Read the model definition and answer for the solid it produces. Units are mm, in the model's axes. Face numbers are marked on the shaded views. A direction names the side the tool comes from. Round coordinates to 2 decimals unless told otherwise and drop trailing zeros. Order: outer loops, then holes, each group sorted by start corner. A loop starts at its lowest first (then second) coordinate and runs counter-clockwise, first axis right, second up. Notation, with made-up numbers: (-24, 36.25) -> (12, 36.25) arc R17 ccw to (12, 67.25) -> close; hole circle Ø4 at (80.25, 17.25). An arc over 180 degrees is marked (long way). One line per item, written item: value. Start each with the question number.
1. Section C-C (z = 11.5) is taken. Give the vertices of the cut face in (x, y).
2. Flat-ended cylindrical pins translate along their axes: pin 1 Ø4.5 at (x, y) = (0, 10.5) entering from -Z; pin 2 Ø4.5 at (x, z) = (-3, 17.5) entering from -Y; pin 3 Ø4.5 at (x, z) = (-1.5, 7.5) entering from +Y. Find the tip coordinate at first contact, or state that the pin passes through.
3. Consider line 1 (X direction, y = 10.5, z = 35.05) (3 decimals); line 2 (Z direction, x = -7, y = -11.5); line 3 (Y direction, x = -0.25, z = 19). Determine where each line is inside the solid, lowest interval first.
4. Section B-B (x = 0) is taken. Give the vertices of the cut face in (y, z) (3 decimals).
5. Section A-A (y = 10.5) is taken. Give the vertices of the cut face in (x, z) (3 decimals), then the cut area to 3 significant figures.
6. For the marked faces 1, 2, 3 and 4, determine the directions among +Z, -Z, +X, -X, +Y, -Y from which every point of the face is accessible in a straight line to the end or side of a thin tool.
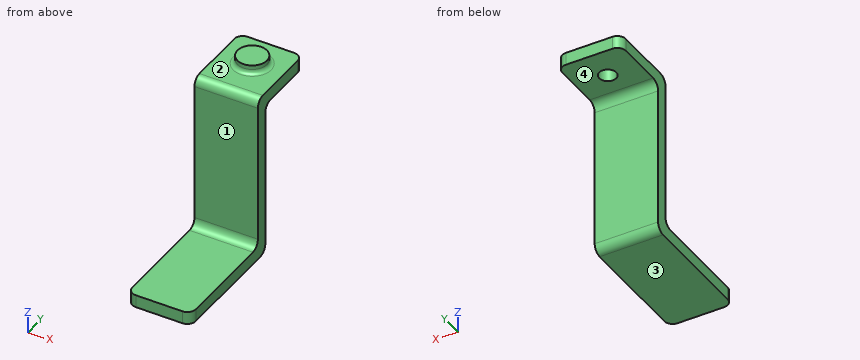
from build123d import *

# Parameters (mm, degrees)
EXTRUDE_1_DEPTH      = 7.5
EXTRUDE_1_DEPTH_BACK = 7.5
FILLET_1_R           = 2
SKETCH_2_R           = 3.5
EXTRUDE_3_DEPTH      = 2
SKETCH_4_R           = 2.025
CUT_EXTRUDE_1_DEPTH  = 4
FILLET_2_R           = 1


with BuildPart() as part:
    # Sketch 1 → Extrude 1 (new, two sides: drawn at the far end of the back side and taken through both)
    with BuildSketch(Plane(origin=(0, 0, 0), x_dir=(0, 0, -1), z_dir=(1, 0, 0)).offset(-EXTRUDE_1_DEPTH_BACK)):
        Polygon((-34, 18), (-34, 3), (3, 3), (3, -27), (0, -27), (0, 0), (-37, 0), (-37, 18), align=None)
    extrude(amount=EXTRUDE_1_DEPTH + EXTRUDE_1_DEPTH_BACK)

    # Fillet 1
    fillet_1_edges = [part.edges().sort_by_distance(p)[0] for p in [
        (0, 3, 34),
        (0, 3, -3),
        (0, 0, 0),
        (0, 0, 37),
        (-7.5, -27, -1.5),
        (7.5, 18, 35.5),
        (7.5, -27, -1.5),
        (-7.5, 18, 35.5),
    ]]
    fillet(fillet_1_edges, radius=FILLET_1_R)

    # Sketch 2 → Extrude 3 (add)
    with BuildSketch(Plane.XY.offset(37)):
        with Locations((0, 10.5)):
            Circle(SKETCH_2_R)
    extrude(amount=EXTRUDE_3_DEPTH)

    # Sketch 4 → Cut-Extrude 1 (cut)
    with BuildSketch(Plane(origin=(0, 0, 34), x_dir=(-1, 0, 0), z_dir=(0, 0, -1))):
        with Locations(Location((0, 10.5, 0), (0, 0, 90))):
            Circle(SKETCH_4_R)
    extrude(amount=-CUT_EXTRUDE_1_DEPTH, mode=Mode.SUBTRACT)

    # Fillet 2
    fillet_2_edges = [part.edges().sort_by_distance(p)[0] for p in [
        (-3.5, 10.5, 37),
    ]]
    fillet(fillet_2_edges, radius=FILLET_2_R)


solid = part.part
Answer:
1. outline: (-7.5, 0) -> (7.5, 0) -> (7.5, 3) -> (-7.5, 3) -> close
2. pin 1: z = 34
2. pin 2: y = 0
2. pin 3: y = 3
3. line 1: -7.5 to -2.025, 2.025 to 7.5
3. line 2: -3 to 0
3. line 3: 0 to 3
4. outline: (-27, -3) -> (1, -3) arc R2 ccw to (3, -1) -> (3, 32) arc R2 cw to (5, 34) -> (8.475, 34) -> (8.475, 38) -> (12.525, 38) -> (12.525, 34) -> (18, 34) -> (18, 37) -> (15, 37) arc R1 cw to (14, 38) -> (14, 39) -> (7, 39) -> (7, 38) arc R1 cw to (6, 37) -> (2, 37) arc R2 ccw to (0, 35) -> (0, 2) arc R2 cw to (-2, 0) -> (-27, 0) -> close
5. outline: (-7.5, 34) -> (-2.025, 34) -> (-2.025, 38) -> (2.025, 38) -> (2.025, 34) -> (7.5, 34) -> (7.5, 37) -> (4.5, 37) arc R1 cw to (3.5, 38) -> (3.5, 39) -> (-3.5, 39) -> (-3.5, 38) arc R1 cw to (-4.5, 37) -> (-7.5, 37) -> close
5. area: 43.2 mm^2
6. face 1: +Z, +X, -X, -Y
6. face 2: +Z
6. face 3: -Z, +X, -X, +Y, -Y
6. face 4: -Z, +X, -X, +Y
